The listing builds one solid part. Answer for the finished solid, in the listing's coordinates (mm). Give positions to 0.01 mm unless a question says otherwise; leave off trailing zeros. Order: outer loops, then holes, each group sorted by start corner. A loop starts at its lowest first (then second) coordinate and runs counter-clockwise, first axis right, second up. Notation, with made-up numbers: (64, 12) -> (113, 12) arc R24 cw to (113, 44) -> close; hole circle Ø7 at (42.5, 68). An arc over 180 degrees is marked (long way). One line per question, with ' | ' between items. Start each with the question number.
```python
from build123d import *

# Parameters (mm, degrees)
F0_R     = 8.25
F0_R_2   = 30
F1_DEPTH = 20
F2_SIZE  = 6
F3_SIZE  = 1


with BuildPart() as f1:
    # F0 (on Front) → F1 (new body)
    with BuildSketch(Plane.XZ):
        with BuildLine():
            Line((-126, -50), (76, -50))
            ThreePointArc((76, -50), (111.355339, -35.355339), (126, 0))
            ThreePointArc((126, 0), (111.355339, 35.355339), (76, 50))
            Line((76, 50), (-126, 50))
            Line((-126, 50), (-126, -50))
        make_face()
        with Locations((-108, -32)):
            Circle(F0_R, mode=Mode.SUBTRACT)
        with Locations((12, -32)):
            Circle(F0_R, mode=Mode.SUBTRACT)
        with Locations((-108, 32)):
            Circle(F0_R, mode=Mode.SUBTRACT)
        with Locations((76, 0)):
            Circle(F0_R_2, mode=Mode.SUBTRACT)
        with Locations((12, 32)):
            Circle(F0_R, mode=Mode.SUBTRACT)
    extrude(amount=F1_DEPTH)

    # F2
    f2_edges = [f1.edges().sort_by_distance(p)[0] for p in [
        (46, -20, 0),
        (46, 0, 0),
    ]]
    chamfer(f2_edges, length=F2_SIZE)

    # F3
    f3_edges = [f1.edges().sort_by_distance(p)[0] for p in [
        (-116.25, -20, -32),
        (-116.25, -20, 32),
        (3.75, -20, -32),
        (3.75, -20, 32),
        (-25, -20, -50),
        (-126, -20, 0),
        (-25, -20, 50),
        (126, -20, 0),
        (-126, -10, -50),
        (-126, 0, 0),
        (-25, 0, -50),
        (-25, 0, 50),
        (-126, -10, 50),
        (-116.25, 0, -32),
        (-116.25, 0, 32),
        (3.75, 0, -32),
        (3.75, 0, 32),
        (126, 0, 0),
    ]]
    chamfer(f3_edges, length=F3_SIZE)


solid = f1.part
```
(1) Determine the mould class of faces 1 (the face through (-23, -10, 50)), 2 (the face through (-26, -10, -50)), 3 (the face through (-126, -10, 1)), 4 (the face through (15.807, -9.874, -39.319)) for opening direction Z: pulls with the +Z half, pulls with the -Z half, needs draft (parallel to the pull), parting line crosses it, or undercut.
(2) Given P1, Ø12, axis at x = 6.5, z = -4, coming from the +Y side, flat-ended and moving along its own axis, determine where the tip first touches the part or whether it passes through.
(3) The part is cut by section B-B on y = -3.25. Determine the outline of the cut face in (x, z), plus the area to 3 significant figures.
(4) Consider line 1 (Z direction, x = -108, y = -14.5); line 2 (X direction, y = -8.5, z = -1.5); line 3 (Z direction, x = 76, y = -8.5). Determine where each line is inside the solid, lowest interval first.
(5) The part is cut by section A-A on x = -108. Determine the outline of the cut face in (y, z), plus the area to 3 significant figures.
Result sheet:
1) face 1: pulls with the +Z half | face 2: pulls with the -Z half | face 3: needs draft | face 4: undercut
2) P1: stops at y = 0
3) outline: (-126, -49) -> (-125, -50) -> (76, -50) arc R50 ccw to (76, 50) -> (-125, 50) -> (-126, 49) -> close; hole circle Ø16.5 at (-108, -32); hole circle Ø16.5 at (-108, 32); hole circle Ø16.5 at (12, -32); hole circle Ø16.5 at (12, 32); hole circle Ø65.5 at (76, 0) | area: 19,900 mm^2
4) line 1: z = -50 to -40.25, -23.75 to 23.75, 40.25 to 50 | line 2: x = -126 to 46.04, 105.96 to 125.98 | line 3: z = -50 to -30, 30 to 50
5) outline: (-20, -49) -> (-19, -50) -> (-1, -50) -> (0, -49) -> (0, -41.25) -> (-1, -40.25) -> (-19, -40.25) -> (-20, -41.25) -> close; (-20, -22.75) -> (-19, -23.75) -> (-1, -23.75) -> (0, -22.75) -> (0, 22.75) -> (-1, 23.75) -> (-19, 23.75) -> (-20, 22.75) -> close; (-20, 41.25) -> (-19, 40.25) -> (-1, 40.25) -> (0, 41.25) -> (0, 49) -> (-1, 50) -> (-19, 50) -> (-20, 49) -> close | area: 1,330 mm^2
